```python
from build123d import *

# Parameters (mm, degrees)
SKETCH_W     = 30
SKETCH_H     = 30
PAD_DEPTH    = 7
SKETCH001_W  = 10
SKETCH001_H  = 8.1
PAD001_DEPTH = 1.5
SKETCH002_R  = 3.1
POCKET_DEPTH = 7.001
CHAMFER_SIZE = 2


with BuildPart() as part:
    # Sketch → Pad (new body)
    with BuildSketch(Plane.XY):
        Rectangle(SKETCH_W, SKETCH_H)
    extrude(amount=PAD_DEPTH)

    # Sketch001 (on Face6 of Pad) → Pad001 (join)
    with BuildSketch(Plane.XY.offset(7)):
        with Locations((-10, 0)):
            Rectangle(SKETCH001_W, SKETCH001_H)
        with Locations((10, 0)):
            Rectangle(SKETCH001_W, SKETCH001_H)
    extrude(amount=PAD001_DEPTH)

    # Sketch002 (on Face5 of Pad001) → Pocket (cut, through all)
    with BuildSketch(Plane.XY.offset(7)):
        Circle(SKETCH002_R)
    extrude(amount=-POCKET_DEPTH, mode=Mode.SUBTRACT)

    # Chamfer
    chamfer_edges = [part.edges().sort_by_distance(p)[0] for p in [
        (15, 0, 0),
        (0, -15, 0),
        (-15, 0, 0),
        (0, 15, 0),
    ]]
    chamfer(chamfer_edges, length=CHAMFER_SIZE)


solid = part.part
```
Part model, mm, in its own coordinate system. A direction names the side the tool comes from. Coordinates: 2 decimals unless noted, no trailing zeros. Order: outer loops, then holes, each group sorted by start corner. A loop starts at its lowest first (then second) coordinate and runs counter-clockwise, first axis right, second up. Notation, with made-up numbers: (-1.5, 0) -> (45.5, 0) arc R15 cw to (45.5, 9) -> close; hole circle Ø5 at (71, 69). An arc over 180 degrees is marked (long way). Put each result on its own line as item: value. Start each with the question number.
(1) Probe line 1 along Y through (x, z) = (0, 4.75); line 2 along Z through (x, y) = (8.75, 4.75); line 3 along Y through (x, z) = (1, 1). List the from-to ranges inside material, lowest first. Write a range as [from, to].
(2) Band-saw the part on A-A (x = 0). Give the cut face in (y, z).
(3) Band-saw the part on B-B (y = 0). Give the cut face in (x, z), then the cut area to 3 significant figures.
(4) Pin check, flat tip, straight feed: pin 1 Ø0.8 at (x, z) = (8.5, 8) entering from +Y. Stop position of the tip, or through.
(5) Which spindle directions (+Z, -Z, +X, -X, +Y, -Y) get a long thin tool onto all of the face, cutting with end or side? Do faces 4 (the face through (-10, 4.05, 8)), 5 (the face through (-10, -4.05, 8)), 6 (the face through (-3, 3, 0)), 7 (the face through (0, -14, 1)), 8 (the face through (5, 0, 8)). Say none if no direction does.
(6) Band-saw the part on D-D (y = -7). Give the cut face in (x, z), then the cut area to 3 significant figures.
(7) Band-saw the part on C-C (z = 4). Give the cut face in (x, y).
(8) Mould opens along X. For faces 1 (the face through (-5, 0, 8)), 2 (the face through (0, -15, 4)), 3 (the face through (14, 0, 1)) say: pulls with the +X half, pulls with the -X half, needs draft (parallel to the pull), parting line crosses it, or undercut.
Determined:
1. line 1: y = [-15, -3.1], [3.1, 15]
1. line 2: z = [0, 7]
1. line 3: y = [-14, -2.93], [2.93, 14]
2. outline: (-15, 2) -> (-13, 0) -> (-3.1, 0) -> (-3.1, 7) -> (-15, 7) -> close; (3.1, 0) -> (13, 0) -> (15, 2) -> (15, 7) -> (3.1, 7) -> close
3. outline: (-15, 2) -> (-13, 0) -> (-3.1, 0) -> (-3.1, 7) -> (-5, 7) -> (-5, 8.5) -> (-15, 8.5) -> close; (3.1, 0) -> (13, 0) -> (15, 2) -> (15, 8.5) -> (5, 8.5) -> (5, 7) -> (3.1, 7) -> close
3. area: 193 mm²
4. pin 1: stops at y = 4.05
5. face 4: +Z, +X, -X, +Y
5. face 5: +Z, +X, -X, -Y
5. face 6: -Z, +X, -X, +Y, -Y
5. face 7: -Z, +X, -X, -Y
5. face 8: +Z, +Y, -Y
6. outline: (-15, 2) -> (-13, 0) -> (13, 0) -> (15, 2) -> (15, 7) -> (-15, 7) -> close
6. area: 206 mm²
7. outline: (-15, -15) -> (15, -15) -> (15, 15) -> (-15, 15) -> close; hole circle Ø6.2 at (0, 0)
8. face 1: undercut
8. face 2: needs draft
8. face 3: pulls with the +X half
